The model under review builds one solid part; all positions refer to its coordinate system, in mm. A direction names the side the tool comes from. Coordinates: 2 decimals unless noted, no trailing zeros. Write each loop counter-clockwise with the first axis right and the second up, starting at its lowest first coordinate (ties: lowest second). Pieces come first, ordered by that corner, then holes. Notation, with made-up numbers: (62.5, 38.5) - (84.5, 38.5) arc R17 ccw to (84.5, 45.5) - close; hole circle Ø5 at (-5.75, 84.25). An arc over 180 degrees is marked (long way). Put each result on its own line as item: value.
from build123d import *

# Parameters (mm, degrees)
CROQUIS1_R              = 6.35
SALIENTE_EXTRUIR1_DEPTH = 117
CROQUIS2_R              = 6.35
SALIENTE_EXTRUIR2_DEPTH = 14
CROQUIS3_R              = 6.35
CORTAR_EXTRUIR1_DEPTH   = 3
CROQUIS4_R              = 25.644678888
CROQUIS4_R_2            = 9.5
CORTAR_EXTRUIR2_DEPTH   = 10
CORTAR_EXTRUIR2_DRAFT   = -42
CROQUIS5_R              = 21.393004687
CROQUIS5_R_2            = 9.5
CORTAR_EXTRUIR3_DEPTH   = 10
CORTAR_EXTRUIR3_DRAFT   = -42
SALIENTE_EXTRUIR3_DEPTH = 14
CORTAR_EXTRUIR4_START   = -3
CROQUIS7_R              = 6.35
CORTAR_EXTRUIR4_DEPTH   = 3
CROQUIS9_R              = 21.176137587
CROQUIS9_R_2            = 9.5
CORTAR_EXTRUIR5_DEPTH   = 3
CORTAR_EXTRUIR5_DRAFT   = -42
REDONDEO1_R             = 0.5


with BuildPart() as part:
    # Croquis1 → Saliente-Extruir1 (new body)
    with BuildSketch(Plane.XY):
        Circle(CROQUIS1_R)
    extrude(amount=-SALIENTE_EXTRUIR1_DEPTH)

    # Croquis2 → Saliente-Extruir2 (add)
    with BuildSketch(Plane.XY):
        Polygon((10.969655115, 0), (5.484827557, 9.5), (-5.484827557, 9.5), (-10.969655115, 0), (-5.484827557, -9.5), (5.484827557, -9.5), align=None)
        Circle(CROQUIS2_R, mode=Mode.SUBTRACT)
    extrude(amount=-SALIENTE_EXTRUIR2_DEPTH)

    # Croquis3 → Cortar-Extruir1 (cut)
    with BuildSketch(Plane.XY):
        Polygon((10.969655115, 0), (5.484827557, 9.5), (-5.484827557, 9.5), (-10.969655115, 0), (-5.484827557, -9.5), (5.484827557, -9.5), align=None)
        Circle(CROQUIS3_R, mode=Mode.SUBTRACT)
    extrude(amount=-CORTAR_EXTRUIR1_DEPTH, mode=Mode.SUBTRACT)


with BuildPart() as cortar_extruir2_tool:
    # Croquis4 → Cortar-Extruir2 (with draft: the straight prism first)
    with BuildSketch(Plane.XY.offset(-3)):
        Circle(CROQUIS4_R)
        Circle(CROQUIS4_R_2, mode=Mode.SUBTRACT)
    extrude(amount=-CORTAR_EXTRUIR2_DEPTH)
    # Cortar-Extruir2: the draft: its side faces are tilted about the plane it starts from
    cortar_extruir2_sides = [cortar_extruir2_tool.faces().sort_by_distance(p)[0] for p in [
        (-25.644678888, 0, -8),
        (-9.5, 0, -8),
    ]]
    draft(cortar_extruir2_sides, Plane.XY.offset(-3), CORTAR_EXTRUIR2_DRAFT)


with BuildPart() as part_1:
    add(part.part)

    # Cortar-Extruir2: cut by cortar_extruir2_tool
    add(cortar_extruir2_tool.part, mode=Mode.SUBTRACT)


with BuildPart() as cortar_extruir3_tool:
    # Croquis5 → Cortar-Extruir3 (with draft: the straight prism first)
    with BuildSketch(Plane(origin=(0, 0, -14), x_dir=(-1, 0, 0), z_dir=(0, 0, -1))):
        Circle(CROQUIS5_R)
        Circle(CROQUIS5_R_2, mode=Mode.SUBTRACT)
    extrude(amount=-CORTAR_EXTRUIR3_DEPTH)
    # Cortar-Extruir3: the draft: its side faces are tilted about the plane it starts from
    cortar_extruir3_sides = [cortar_extruir3_tool.faces().sort_by_distance(p)[0] for p in [
        (21.393004687, 0, -9),
        (9.5, 0, -9),
    ]]
    draft(cortar_extruir3_sides, Plane(origin=(0, 0, -14), x_dir=(-1, 0, 0), z_dir=(0, 0, -1)), CORTAR_EXTRUIR3_DRAFT)


with BuildPart() as part_2:
    add(part_1.part)

    # Cortar-Extruir3: cut by cortar_extruir3_tool
    add(cortar_extruir3_tool.part, mode=Mode.SUBTRACT)

    # Croquis6 → Saliente-Extruir3 (add)
    with BuildSketch(Plane(origin=(0, 0, -117), x_dir=(-1, 0, 0), z_dir=(0, 0, -1))):
        Polygon((10.969655115, 0), (5.484827557, 9.5), (-5.484827557, 9.5), (-10.969655115, 0), (-5.484827557, -9.5), (5.484827557, -9.5), align=None)
    extrude(amount=-SALIENTE_EXTRUIR3_DEPTH)

    # Croquis7 → Cortar-Extruir4 (cut)
    with BuildSketch(Plane(origin=(0, 0, -117), x_dir=(-1, 0, 0), z_dir=(0, 0, -1)).offset(CORTAR_EXTRUIR4_START)):
        Polygon((10.969655115, 0), (5.484827557, 9.5), (-5.484827557, 9.5), (-10.969655115, 0), (-5.484827557, -9.5), (5.484827557, -9.5), align=None)
        with Locations(Location((0, 0, 0), (0, 0, 180))):
            Circle(CROQUIS7_R, mode=Mode.SUBTRACT)
    extrude(amount=CORTAR_EXTRUIR4_DEPTH, mode=Mode.SUBTRACT)


with BuildPart() as cortar_extruir5_tool:
    # Croquis9 → Cortar-Extruir5 (with draft: the straight prism first)
    with BuildSketch(Plane(origin=(0, 0, -114), x_dir=(-1, 0, 0), z_dir=(0, 0, -1))):
        Circle(CROQUIS9_R)
        Circle(CROQUIS9_R_2, mode=Mode.SUBTRACT)
    extrude(amount=-CORTAR_EXTRUIR5_DEPTH)
    # Cortar-Extruir5: the draft: its side faces are tilted about the plane it starts from
    cortar_extruir5_sides = [cortar_extruir5_tool.faces().sort_by_distance(p)[0] for p in [
        (21.176137587, 0, -112.5),
        (9.5, 0, -112.5),
    ]]
    draft(cortar_extruir5_sides, Plane(origin=(0, 0, -114), x_dir=(-1, 0, 0), z_dir=(0, 0, -1)), CORTAR_EXTRUIR5_DRAFT)


with BuildPart() as part_3:
    add(part_2.part)

    # Cortar-Extruir5: cut by cortar_extruir5_tool
    add(cortar_extruir5_tool.part, mode=Mode.SUBTRACT)

    # Redondeo1
    redondeo1_edges = [part_3.edges().sort_by_distance(p)[0] for p in [
        (-6.35, 0, 0),
    ]]
    fillet(redondeo1_edges, radius=REDONDEO1_R)


solid = part_3.part
1. Machinability: for faces 1 (the conical face through (-4.904, -8.543, -13.611)), 2 (the flat face through (2, -6.2, -3)), 3 (the flat face through (8.266, -4.684, -108.577)), 4 (the conical face through (4.95, -8.52, -13.61)), 5 (the conical face through (4.904, 8.543, -13.611)), which of the approach directions +Z, -Z, +X, -X, +Y, -Y give a long, thin tool a straight path to every point of the face, cutting with its end or side? Answer none if there is none.
Determined:
face 1: -X, -Y
face 2: +Z
face 3: +Z, -Z, +X, -Y
face 4: +X, -Y
face 5: +X, +Y
2. The part is to be moulded in two halves that separate along Z. For faces 6 (the cylindrical face through (-1.38, -6.2, -1.73)), 7 (the conical face through (9.85, 0.02, -13.61)), 8 (the conical face through (4.95, -8.52, -113.61)), say which applies: +Z half, -Z half, draft (parallel to the pull), parting line (faces both ways), or undercut.
Determined:
face 6: draft
face 7: undercut
face 8: -Z half
3. Consider section A-A on z = -27. State the section outline as (x, y) points.
Determined:
outline: circle Ø12.7 at (0, 0)
4. For pin 1 Ø6 at (y, z) = (5, -59) entering from -X; pin 2 Ø5 at (x, z) = (3.5, -74.5) entering from +Y; pin 3 Ø1 at (y, z) = (-4.5, -96.5) entering from +X, all flat-tipped, find the tip position at first contact; note any pin that passes through.
Determined:
pin 1: stops at x = -6.03
pin 2: stops at y = 6.27
pin 3: stops at x = 4.93
5. To check wall thickness, follow probe 1 along Z at (x, y) = (-8.5, -2); probe 2 along Y at (x, z) = (0, -94); probe 3 along Y at (x, z) = (-2.5, -71). State the ranges of each line that lie inside material, in increasing order.
Determined:
probe 1: z = -114 to -103, -14 to -3
probe 2: y = -6.35 to 6.35
probe 3: y = -5.84 to 5.84
